Here's how the part is built. I have some questions about the finished solid (model axes, mm). Face numbers are marked on the shaded views. A direction names the side the tool comes from. Coordinates: 2 decimals unless noted, no trailing zeros. Write each loop counter-clockwise with the first axis right and the second up, starting at its lowest first coordinate (ties: lowest second). Pieces come first, ordered by that corner, then holes.
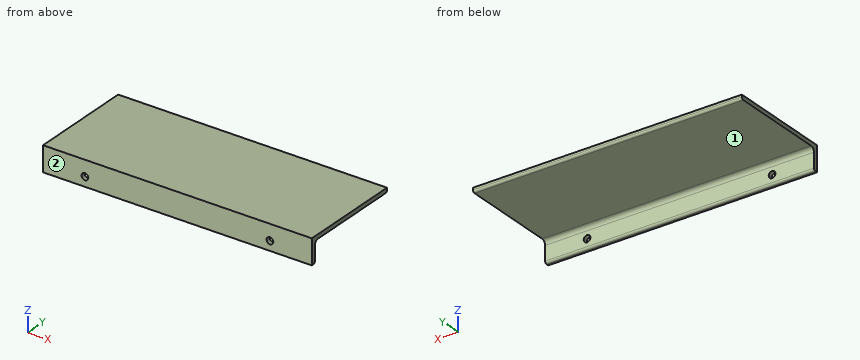
```python
from build123d import *

# Parameters (mm, degrees)
BOSS_EXTRUDE1_DEPTH = 128.27
FILLET1_R           = 1
FILLET2_R           = 2
SKETCH2_R           = 1.6
CUT_EXTRUDE1_DEPTH  = 188.253444223


with BuildPart() as part:
    # Sketch1 → Boss-Extrude1 (new body)
    with BuildSketch(Plane(origin=(0, 0, 0), x_dir=(0, 0, -1), z_dir=(1, 0, 0))):
        Polygon((-127.697531195, -39.21530097), (-127.697531195, -89.21530097), (-115.697531195, -89.21530097), (-115.697531195, -87.21530097), (-125.697531195, -87.21530097), (-125.697531195, -39.21530097), align=None)
    extrude(amount=BOSS_EXTRUDE1_DEPTH)

    # Fillet1
    fillet1_edges = [part.edges().sort_by_distance(p)[0] for p in [
        (64.135, -39.21530097, 125.697531195),
        (64.135, -87.21530097, 115.697531195),
    ]]
    fillet(fillet1_edges, radius=FILLET1_R)

    # Fillet2
    fillet2_edges = [part.edges().sort_by_distance(p)[0] for p in [
        (64.135, -87.21530097, 125.697531195),
    ]]
    fillet(fillet2_edges, radius=FILLET2_R)

    # Sketch2 → Cut-Extrude1 (cut, through all)
    with BuildSketch(Plane(origin=(0, -87.21530097, 0), x_dir=(1, 0, 0), z_dir=(0, 1, 0))):
        with Locations(Location((20, -120.197531195, 0), (0, 0, 270))):
            Circle(SKETCH2_R)
        with Locations(Location((108.27, -120.197531195, 0), (0, 0, 270))):
            Circle(SKETCH2_R)
    extrude(amount=-CUT_EXTRUDE1_DEPTH, mode=Mode.SUBTRACT)


solid = part.part
```
1) Will these pins go through, and if not, where does the flat tip stop? pin 1 (5 mm diameter, centred on y = -80, z = 122.5, fed in from -X); pin 2 (22.5 mm diameter, centred on x = 52, y = -68, fed in from -Z); pin 3 (5 mm diameter, centred on x = 108.27, z = 120.2, fed in from +Y); pin 4 (5.5 mm diameter, centred on x = 50, z = 121.5, fed in from +Y).
Values follow:
pin 1: passes through
pin 2: stops at z = 125.7
pin 3: stops at y = -87.22
pin 4: stops at y = -87.14
2) Imagine slicing it at C-C on y = -43.5. Please give me the cut outline in (x, z).
Values follow:
outline: (0, 125.7) - (128.27, 125.7) - (128.27, 127.7) - (0, 127.7) - close
3) Imagine slicing it at A-A on x = 108.27. Please give me the cut outline in (y, z), then the cut area to 3 significant figures.
Values follow:
outline: (-89.22, 115.7) - (-88.22, 115.7) arc R1 ccw to (-87.22, 116.7) - (-87.22, 118.6) - (-89.22, 118.6) - close; (-89.22, 121.8) - (-87.22, 121.8) - (-87.22, 123.7) arc R2 cw to (-85.22, 125.7) - (-40.22, 125.7) arc R1 ccw to (-39.22, 126.7) - (-39.22, 127.7) - (-89.22, 127.7) - close
area: 114 mm2
4) On a 3-axis mill with a long thin cutter (end or side, diameter ignored), from which of +Z, -Z, +X, -X, +Y, -Y can I reach the whole of each face in a straight line? I mean the marked faces 1 and 2. Say none if no direction works.
Values follow:
face 1: -Z, +X, -X, +Y
face 2: +Z, -Z, +X, -X, -Y
5) I need wall thicknesses on probe 1 along Z at (x, y) = (108.27, -88.25); probe 2 along Z at (x, y) = (77, -69.5); probe 3 along Y at (x, z) = (86.5, 122.5). Which ranges of each line are inside material? Lowest first, please.
Values follow:
probe 1: z = 115.7 to 118.6, 121.8 to 127.7
probe 2: z = 125.7 to 127.7
probe 3: y = -89.22 to -87.22
6) Imagine slicing it at B-B on x = 27. Please give me the cut outline in (y, z).
Values follow:
outline: (-89.22, 115.7) - (-88.22, 115.7) arc R1 ccw to (-87.22, 116.7) - (-87.22, 123.7) arc R2 cw to (-85.22, 125.7) - (-40.22, 125.7) arc R1 ccw to (-39.22, 126.7) - (-39.22, 127.7) - (-89.22, 127.7) - close
